Verification items for the finished model (mm, model axes). A direction names the side the tool comes from. Coordinates: 2 decimals unless noted, no trailing zeros. Loops run counter-clockwise (first coordinate to the right, second up) from the corner with the lowest first, then second, coordinate; pieces in that order, holes last. Notation, with made-up numbers: (13, 25.5) -> (22, 25.5) arc R32 cw to (22, 61.5) -> close; hole circle Ø4 at (72, 18.5). An arc over 180 degrees is marked (long way). Answer as a JSON object with one key per item and string values. Group by question number.
Q1. Set-up check for faces 1 (the flat face through (2, 4, 0)), 2 (the flat face through (10, 3.2, -146)): record each of +Z, -Z, +X, -X, +Y, -Y from which the full face is reachable in a straight line by a thin tool's end or side.
Q2. Cross-section at A-A on z = -225. Record the boundary of the cut face in (x, y).
Q3. Gauge pin test, flat ends, axial feed: pin 1 Ø3 at (x, z) = (9.6, -8) entering from +Y (3 decimals); pin 2 Ø6 at (x, z) = (11, -106.5) entering from +Y; pin 3 Ø5 at (y, z) = (9.6, -216) entering from +X; pin 4 Ø4.5 at (x, z) = (9.6, -216) entering from -Y. Record the tip position at first contact, or that the pin passes through.
Q4. Scan lines: L1, parallel to Y at x = 1.05, z = -8; L2, parallel to X at y = 11.75, z = -226.5. Record each from-to range of solid material in increasing order.
```python
from build123d import *

# Parameters (mm, degrees)
SKETCH1_W                      = 16
SKETCH1_H                      = 288
BOSS_EXTRUDE1_DEPTH            = 16
SKETCH2_W                      = 12.8
SKETCH2_H                      = 12.8
CUT_EXTRUDE1_DEPTH             = 289
F_3_7_3_7_DIAMETER_HOLE1_D     = 3.7
F_3_7_3_7_DIAMETER_HOLE1_DEPTH = 16
F_3_7_3_7_DIAMETER_HOLE2_D     = 3.7
F_3_7_3_7_DIAMETER_HOLE2_DEPTH = 16
FILLET1_R                      = 2


with BuildPart() as part:
    # Sketch1 → Boss-Extrude1 (new body)
    with BuildSketch(Plane(origin=(0, 16, 0), x_dir=(1, 0, 0), z_dir=(0, 1, 0))):
        with Locations((8, 144)):
            Rectangle(SKETCH1_W, SKETCH1_H)
    extrude(amount=-BOSS_EXTRUDE1_DEPTH)

    # Sketch2 → Cut-Extrude1 (cut, through all)
    with BuildSketch(Plane(origin=(0, 0, -288), x_dir=(-1, 0, 0), z_dir=(0, 0, -1))):
        with Locations((-9.6, 9.6)):
            Rectangle(SKETCH2_W, SKETCH2_H)
    extrude(amount=-CUT_EXTRUDE1_DEPTH, mode=Mode.SUBTRACT)

    # Ø3.7 (3.7) Diameter Hole1
    with Locations(Plane(origin=(0, 0, 0), x_dir=(-1, 0, 0), z_dir=(0, -1, 0))):
        with Locations((-9.6, 24), (-9.6, 40), (-9.6, 56), (-9.6, 72), (-9.6, 88), (-9.6, 104), (-9.6, 120), (-9.6, 136), (-9.6, 152), (-9.6, 168), (-9.6, 184), (-9.6, 200), (-9.6, 216), (-9.6, 232), (-9.6, 248), (-9.6, 264), (-9.6, 280), (-9.6, 8)):
            Hole(F_3_7_3_7_DIAMETER_HOLE1_D / 2, depth=F_3_7_3_7_DIAMETER_HOLE1_DEPTH)

    # Ø3.7 (3.7) Diameter Hole2
    with Locations(Plane.ZY):
        with Locations((-24, 9.6), (-40, 9.6), (-56, 9.6), (-72, 9.6), (-88, 9.6), (-104, 9.6), (-120, 9.6), (-136, 9.6), (-152, 9.6), (-168, 9.6), (-184, 9.6), (-200, 9.6), (-216, 9.6), (-232, 9.6), (-248, 9.6), (-264, 9.6), (-280, 9.6), (-8, 9.6)):
            Hole(F_3_7_3_7_DIAMETER_HOLE2_D / 2, depth=F_3_7_3_7_DIAMETER_HOLE2_DEPTH)

    # Fillet1
    fillet1_edges = [part.edges().sort_by_distance(p)[0] for p in [
        (1.6, 16, -288),
        (1.6, 16, 0),
        (16, 1.6, -288),
        (16, 1.6, 0),
    ]]
    fillet(fillet1_edges, radius=FILLET1_R)


solid = part.part
```
Computed values:
{
 "1": {"face 1": "+Z, +X, -X, +Y, -Y", "face 2": "+Z, -Z, +X, +Y"},
 "2": {"outline": "(0, 0) -> (16, 0) -> (16, 3.2) -> (3.2, 3.2) -> (3.2, 16) -> (0, 16) -> close"},
 "3": {"pin 1": "passes through", "pin 2": "stops at y = 3.2", "pin 3": "stops at x = 3.2", "pin 4": "stops at y = 0"},
 "4": {"L1": "y = 0 to 7.75, 11.45 to 16", "L2": "x = 0 to 3.2"}
}
